Geometry: final body of the model. Coordinates: model frame, mm. A direction names the side the tool comes from. Give positions to 0.01 mm unless a question says otherwise; leave off trailing zeros. Order: outer loops, then holes, each group sorted by start corner. A loop starts at its lowest first (then second) coordinate and runs counter-clockwise, first axis right, second up. Notation, with made-up numbers: (24.25, -39) - (45.25, -39) arc R17 cw to (45.25, -16) - close; hole circle Ø7 at (26.25, -7.75). An arc over 180 degrees is marked (long way). One line per question, with ' | ' between items. Start each with the question number.
from build123d import *

# Parameters (mm, degrees)
SKETCH1_W           = 51.53
SKETCH1_H           = 30
BOSS_EXTRUDE1_DEPTH = 5
CUT_EXTRUDE1_DEPTH  = 5
FILLET1_R           = 10
CUT_EXTRUDE5_DEPTH  = 10


with BuildPart() as part:
    # Sketch1 → Boss-Extrude1 (new body)
    with BuildSketch(Plane.XY):
        with Locations((2.765, -5)):
            Rectangle(SKETCH1_W, SKETCH1_H)
    extrude(amount=BOSS_EXTRUDE1_DEPTH)

    # Sketch2 → Cut-Extrude1 (cut)
    with BuildSketch(Plane.XY.offset(5)):
        Polygon((13.53, -1.9), (20.865904873, -1.9), (20.865904873, -3.4), (24.265904873, -3.4), (24.265904873, -1.9), (28.53, -1.9), (28.53, 2.5), (24.265904873, 2.5), (24.265904873, 4), (20.865904873, 4), (20.865904873, 2.5), (13.53, 2.5), align=None)
        Polygon((4.13, -5), (4.13, -11.6), (2.63, -11.6), (2.63, -15), (4.13, -15), (4.13, -20), (8.53, -20), (8.53, -15), (10.03, -15), (10.03, -11.6), (8.53, -11.6), (8.53, -5), align=None)
    extrude(amount=-CUT_EXTRUDE1_DEPTH, mode=Mode.SUBTRACT)

    # Fillet1
    fillet1_edges = [part.edges().sort_by_distance(p)[0] for p in [
        (-23, 10, 2.5),
    ]]
    fillet(fillet1_edges, radius=FILLET1_R)

    # Sketch6 → Cut-Extrude5 (cut)
    with BuildSketch(Plane.XY.offset(5)):
        with BuildLine():
            Line((-16.500870191, -3.314520992), (-10.500870191, -3.314520992))
            ThreePointArc((-10.500870191, -3.314520992), (-8.900870191, -4.914520992), (-10.500870191, -6.514520992))
            Line((-10.500870191, -6.514520992), (-16.500870191, -6.514520992))
            ThreePointArc((-16.500870191, -6.514520992), (-18.100870191, -4.914520992), (-16.500870191, -3.314520992))
        make_face()
    extrude(amount=-CUT_EXTRUDE5_DEPTH, mode=Mode.SUBTRACT)


solid = part.part
(1) Pull-direction query (X, two-part tool) for faces 4 (the flat face through (10.03, -13, 3)), 5 (the flat face through (28.53, -11, 2)), 6 (the flat face through (26, 2.5, 3)); classes: +X half, -X half, draft (parallel to the pull), parting line (faces both ways), or undercut.
(2) Cut plane D-D, the plane x = 8. Return the cut outline in (y, z).
(3) Material intervals for line 1 along Y through (x, z) = (25.5, 2.05); line 2 along X through (y, z) = (-16, 2.4); line 3 along X through (y, z) = (-12, 4.2), sorted ascending. Write a range as from..to.
(4) Access query for faces 1 (the flat face through (28.53, 6, 2)), 2 (the cylindrical face through (-8.9, -4.9, 2.5)), 3 (the flat face through (8.53, -8, 3)). Directions: +Z, -Z, +X, -X, +Y, -Y. A direction counts if a zero-diameter tool reaches every point of the face in a straight line with its end or side. Return the directions, or none.
(5) Cut plane A-A, the plane x = 25. Return the cut outline in (y, z).
(6) Contact query for a flat-ended pin moving along its axis: P1, Ø0.8, axis at y = 3, z = 1.5, coming from the -X side. Output: stop coordinate, or through.
(7) Cut plane B-B, the plane y = -17. Return the cut outline in (x, z), plus the area to 3 significant figures.
Results are:
1) face 4: undercut | face 5: +X half | face 6: draft
2) outline: (-5, 0) - (10, 0) - (10, 5) - (-5, 5) - close
3) line 1: -20..-1.9, 2.5..10 | line 2: -23..4.13, 8.53..28.53 | line 3: -23..2.63, 10.03..28.53
4) face 1: +Z, -Z, +X, +Y, -Y | face 2: +Z, -Z | face 3: +Z, -Z, -Y
5) outline: (-20, 0) - (-1.9, 0) - (-1.9, 5) - (-20, 5) - close; (2.5, 0) - (10, 0) - (10, 5) - (2.5, 5) - close
6) P1: x = -22.66
7) outline: (-23, 0) - (4.13, 0) - (4.13, 5) - (-23, 5) - close; (8.53, 0) - (28.53, 0) - (28.53, 5) - (8.53, 5) - close | area: 236 mm2
